from build123d import *

# Parameters (mm, degrees)
MODEL_R             = 1.775
MODEL_W             = 6.86
MODEL_H             = 15
BOSS_EXTRUDE1_DEPTH = 6.6


with BuildPart() as part:
    # Model → Boss-Extrude1 (new body)
    with BuildSketch(Plane.XY):
        with BuildLine():
            Line((213.28, 98.3), (2, 98.3))
            ThreePointArc((2, 98.3), (0.585786438, 97.714213562), (0, 96.3))
            Line((0, 96.3), (0, 2))
            ThreePointArc((0, 2), (0.585786438, 0.585786438), (2, 0))
            Line((2, 0), (213.28, 0))
            ThreePointArc((213.28, 0), (214.694213562, 0.585786438), (215.28, 2))
            Line((215.28, 2), (215.28, 96.3))
            ThreePointArc((215.28, 96.3), (214.694213562, 97.714213562), (213.28, 98.3))
        make_face()
        with Locations((10.310000096, 59.15)):
            Circle(MODEL_R, mode=Mode.SUBTRACT)
        with Locations((204.970000096, 59.15)):
            Circle(MODEL_R, mode=Mode.SUBTRACT)
        with Locations((91.820001761, 55.71)):
            Circle(MODEL_R, mode=Mode.SUBTRACT)
        with Locations((124.08000176, 55.71)):
            Circle(MODEL_R, mode=Mode.SUBTRACT)
        with BuildLine():
            Line((135.316050952, 59.858691011), (171.867952568, 59.858691011))
            ThreePointArc((171.867952568, 59.858691011), (173.409261558, 61.4), (171.867952568, 62.941308989))
            Line((171.867952568, 62.941308989), (135.316050952, 62.941308989))
            ThreePointArc((135.316050952, 62.941308989), (133.774741963, 61.4), (135.316050952, 59.858691011))
        make_face(mode=Mode.SUBTRACT)
        with BuildLine():
            Line((135.316050952, 47.858691011), (171.867952568, 47.858691011))
            ThreePointArc((171.867952568, 47.858691011), (173.409261558, 49.4), (171.867952568, 50.941308989))
            Line((171.867952568, 50.941308989), (135.316050952, 50.941308989))
            ThreePointArc((135.316050952, 50.941308989), (133.774741963, 49.4), (135.316050952, 47.858691011))
        make_face(mode=Mode.SUBTRACT)
        with Locations((91.820001761, 83.92)):
            Rectangle(MODEL_W, MODEL_H, mode=Mode.SUBTRACT)
        with Locations((124.08000176, 83.92)):
            Rectangle(MODEL_W, MODEL_H, mode=Mode.SUBTRACT)
        with Locations((204.970000096, 40.2)):
            Rectangle(MODEL_W, MODEL_H, mode=Mode.SUBTRACT)
        with Locations((204.970000096, 78.1)):
            Rectangle(MODEL_W, MODEL_H, mode=Mode.SUBTRACT)
        with Locations((10.310000096, 40.2)):
            Rectangle(MODEL_W, MODEL_H, mode=Mode.SUBTRACT)
        with Locations((10.310000096, 78.1)):
            Rectangle(MODEL_W, MODEL_H, mode=Mode.SUBTRACT)
        with BuildLine():
            Line((171.867952568, 26.941308989), (135.316050952, 26.941308989))
            ThreePointArc((135.316050952, 26.941308989), (133.774741963, 25.4), (135.316050952, 23.858691011))
            Line((135.316050952, 23.858691011), (171.867952568, 23.858691011))
            ThreePointArc((171.867952568, 23.858691011), (173.409261558, 25.4), (171.867952568, 26.941308989))
        make_face(mode=Mode.SUBTRACT)
        with BuildLine():
            Line((171.867952568, 38.941308989), (135.316050952, 38.941308989))
            ThreePointArc((135.316050952, 38.941308989), (133.774741963, 37.4), (135.316050952, 35.858691011))
            Line((135.316050952, 35.858691011), (171.867952568, 35.858691011))
            ThreePointArc((171.867952568, 35.858691011), (173.409261558, 37.4), (171.867952568, 38.941308989))
        make_face(mode=Mode.SUBTRACT)
    extrude(amount=BOSS_EXTRUDE1_DEPTH)


solid = part.part
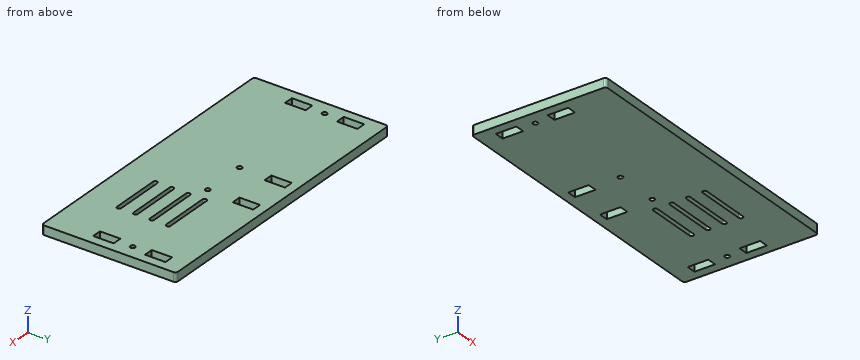
CAD build for the part. Positions are in the model's coordinates, mm. Coordinates: 2 decimals unless noted, no trailing zeros. Loops run counter-clockwise (first coordinate to the right, second up) from the corner with the lowest first, then second, coordinate; pieces in that order, holes last. Notation, with made-up numbers: (-26.5, 18.5) -> (-7.5, 18.5) arc R28 cw to (-7.5, 54.5) -> close; hole circle Ø10 at (59, 3). An arc over 180 degrees is marked (long way). One line per item, written item: value.
1. Slice it at A-A on y = 89. Write the cut outline in (x, z).
Answers:
outline: (0, 0) -> (88.39, 0) -> (88.39, 6.6) -> (0, 6.6) -> close; (95.25, 0) -> (120.65, 0) -> (120.65, 6.6) -> (95.25, 6.6) -> close; (127.51, 0) -> (215.28, 0) -> (215.28, 6.6) -> (127.51, 6.6) -> close
2. Slice it at B-B on x = 142. Write the cut outline in (y, z).
Answers:
outline: (0, 0) -> (23.86, 0) -> (23.86, 6.6) -> (0, 6.6) -> close; (26.94, 0) -> (35.86, 0) -> (35.86, 6.6) -> (26.94, 6.6) -> close; (38.94, 0) -> (47.86, 0) -> (47.86, 6.6) -> (38.94, 6.6) -> close; (50.94, 0) -> (59.86, 0) -> (59.86, 6.6) -> (50.94, 6.6) -> close; (62.94, 0) -> (98.3, 0) -> (98.3, 6.6) -> (62.94, 6.6) -> close
3. Drill centre lines: line 1 (X direction, y = 73, z = 5.5); line 2 (X direction, y = 89, z = 1); line 3 (Y direction, x = 159, z = 2). Where is each one in solid material? Low to high. Write a range as [from, to].
Answers:
line 1: x = [0, 6.88], [13.74, 201.54], [208.4, 215.28]
line 2: x = [0, 88.39], [95.25, 120.65], [127.51, 215.28]
line 3: y = [0, 23.86], [26.94, 35.86], [38.94, 47.86], [50.94, 59.86], [62.94, 98.3]
4. Slice it at C-C on z = 3. Give the number of separate pieces and of enclosed holes in the cut face, and give its area (3 significant figures).
Answers:
separate pieces: 1
enclosed holes: 14
area: 20,000 mm^2
